Geometry check sheet. Reference: the model listing, model coordinates, mm. A direction names the side the tool comes from. Give positions to 0.01 mm unless a question says otherwise; leave off trailing zeros. Write each loop counter-clockwise with the first axis right and the second up, starting at its lowest first coordinate (ties: lowest second). Pieces come first, ordered by that corner, then holes. Notation, with made-up numbers: (25, 29.5) - (66, 29.5) arc R36 cw to (66, 64.5) - close; hole circle Ø10 at (83, 77). An arc over 180 degrees is marked (long way). One line per question, with ' | ' between items. Start each with the question number.
Q1. Gauge pin test, flat ends, axial feed: P1, Ø2, axis at y = 11.5, z = 5, coming from the -X side; P2, Ø10, axis at y = -8.5, z = 31.5, coming from the +X side; P3, Ø2, axis at x = 1, y = 11.5, coming from the +Z side; P4, Ø3, axis at y = 1, z = 18, coming from the -X side. Record the tip position at first contact, or that the pin passes through.
Q2. Section check B-B on z = 3.5. Record the boundary of the cut face in (x, y) (3 decimals), and give its area (3 significant figures).
Q3. Section check C-C on z = 33.5. Record the boundary of the cut face in (x, y).
Q4. Set-up check for faces 5 (the face through (-24, 0, 12)), 6 (the face through (24.112, 0.356, 22.4)), 7 (the face through (25, 0, 12)): record each of +Z, -Z, +X, -X, +Y, -Y from which the full face is reachable in a straight line by a thin tool's end or side.
Q5. Release check for a two-part mould opening along Y. For faces 1 (the face through (10, -5, 12.7)), 2 (the face through (-3.307, 25.184, 6.439)), 3 (the face through (-24.148, 0.356, 22.4)), 4 (the face through (-7.559, -5.796, 5.635)) record: +Y half, -Y half, draft (parallel to the pull), parting line (faces both ways), or undercut.
Q6. Section check A-A on x = 0. Record the boundary of the cut face in (y, z) (3 decimals).
Q7. Thickness scan on L1, parallel to Z at x = 7.5, y = 9; L2, parallel to Y at x = 0, z = 8.25 (3 decimals); L3, parallel to Y at x = -6, z = 10.5. Record the ranges inside material, lowest first. Write a range as [from, to].
```python
from build123d import *

# Parameters (mm, degrees)
SKETCH1_R                     = 25.4
SKETCH1_R_2                   = 9.525
BOSS_EXTRUDE1_DEPTH           = 12.7
CHAMFER1_SIZE                 = 2.54
FILLET1_R                     = 1.27
EXTRUDE_THIN2_DEPTH           = 25.4
EXTRUDE_THIN2_DRAFT           = 2.1
EXTRUDE_THIN2_OTHER_WAY_DEPTH = 2.54


with BuildPart() as part:
    # Sketch1 → Boss-Extrude1 (new body)
    with BuildSketch(Plane.XY):
        Circle(SKETCH1_R)
        Circle(SKETCH1_R_2, mode=Mode.SUBTRACT)
    extrude(amount=BOSS_EXTRUDE1_DEPTH)

    # Chamfer1
    chamfer1_edges = [part.edges().sort_by_distance(p)[0] for p in [
        (-25.4, 0, 12.7),
    ]]
    chamfer(chamfer1_edges, length=CHAMFER1_SIZE)

    # Fillet1
    fillet1_edges = [part.edges().sort_by_distance(p)[0] for p in [
        (-9.525, 0, 12.7),
    ]]
    fillet(fillet1_edges, radius=FILLET1_R)


with BuildPart() as extrude_thin2_tool:
    # Sketch2 → Extrude-Thin2 (with draft: the straight prism first)
    with BuildSketch(Plane.XY.offset(12.7)):
        with BuildLine():
            Line((22.86, 0), (25.4, 0))
            ThreePointArc((25.4, 0), (0, 25.4), (-25.4, 0))
            Line((-25.4, 0), (-22.86, 0))
            ThreePointArc((-22.86, 0), (0, 22.86), (22.86, 0))
        make_face()
    extrude(amount=EXTRUDE_THIN2_DEPTH)
    # Extrude-Thin2: the draft: its side faces are tilted about the plane it starts from
    extrude_thin2_sides = [extrude_thin2_tool.faces().sort_by_distance(p)[0] for p in [
        (24.13, 0, 25.4),
        (0, 25.4, 25.4),
        (-24.13, 0, 25.4),
        (0, 22.86, 25.4),
    ]]
    draft(extrude_thin2_sides, Plane.XY.offset(12.7), EXTRUDE_THIN2_DRAFT)


with BuildPart() as part_1:
    add(part.part)

    # Extrude-Thin2: add extrude_thin2_tool
    add(extrude_thin2_tool.part)

    # Sketch2 → Extrude-Thin2 other way (add)
    with BuildSketch(Plane.XY.offset(12.7)):
        with BuildLine():
            Line((22.86, 0), (25.4, 0))
            ThreePointArc((25.4, 0), (0, 25.4), (-25.4, 0))
            Line((-25.4, 0), (-22.86, 0))
            ThreePointArc((-22.86, 0), (0, 22.86), (22.86, 0))
        make_face()
    extrude(amount=-EXTRUDE_THIN2_OTHER_WAY_DEPTH)


solid = part_1.part
```
Working result:
1) P1: stops at x = -23.13 | P2: passes through | P3: stops at z = 12.7 | P4: stops at x = -25.25
2) outline: circle Ø50.8 at (0, 0); hole circle Ø19.05 at (0, 0) | area: 1,740 mm2
3) outline: (-24.63, 0.76) - (-23.61, 0.76) arc R23.62 cw to (23.61, 0.76) - (24.63, 0.76) arc R24.64 ccw to start
4) face 5: +Z, -X, -Y | face 6: +Z, +X, -X, -Y | face 7: +Z, +X, -Y
5) face 1: draft | face 2: parting line | face 3: -Y half | face 4: undercut
6) outline: (-25.4, 0) - (-9.525, 0) - (-9.525, 11.43) arc R1.27 ccw to (-10.795, 12.7) - (-22.86, 12.7) - (-25.4, 10.16) - close; (9.525, 0) - (25.4, 0) - (25.4, 12.7) - (24.469, 38.1) - (23.791, 38.1) - (22.86, 12.7) - (10.795, 12.7) arc R1.27 ccw to (9.525, 11.43) - close
7) L1: z = [0, 12.7] | L2: y = [-25.4, -9.525], [9.525, 25.4] | L3: y = [-24.33, -7.4], [7.4, 24.68]
